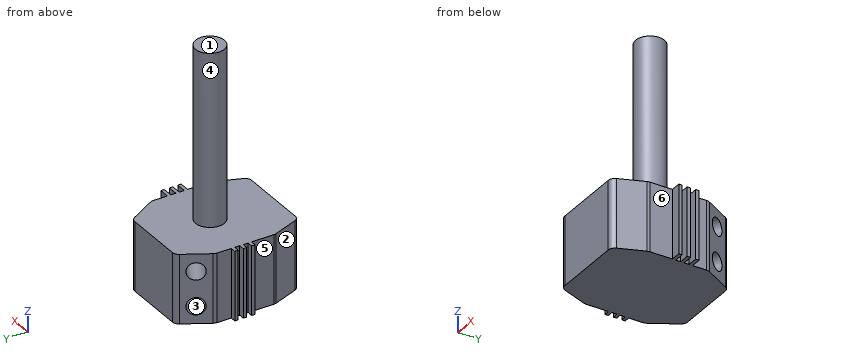
```python
from build123d import *

# Parameters (mm, degrees)
BOSS_EXTRUDE1_DEPTH = 20
SKETCH2_R           = 4.175
BOSS_EXTRUDE2_DEPTH = 50
SKETCH3_R           = 2.5
CUT_EXTRUDE1_DEPTH  = 20
SKETCH4_R           = 2.5
CUT_EXTRUDE2_DEPTH  = 20
SKETCH5_W           = 20
SKETCH5_H           = 1
BOSS_EXTRUDE3_DEPTH = 3


with BuildPart() as part:
    # Sketch1 → Boss-Extrude1 (new body)
    with BuildSketch(Plane.XY):
        with BuildLine():
            Line((7.995487969, -56.473761751), (-9.363697209, -56.473761751))
            ThreePointArc((-9.363697209, -56.473761751), (-10.367550845, -56.743941564), (-11.100183493, -57.481483874))
            Line((-11.100183493, -57.481483874), (-15.206075193, -64.666794349))
            ThreePointArc((-15.206075193, -64.666794349), (-15.402588207, -65.145736355), (-15.469588909, -65.659072225))
            Line((-15.469588909, -65.659072225), (-15.469588909, -82.177343211))
            ThreePointArc((-15.469588909, -82.177343211), (-15.435979311, -82.54245797), (-15.336280121, -82.895301369))
            Line((-15.336280121, -82.895301369), (-12.59092286, -90.03323025))
            ThreePointArc((-12.59092286, -90.03323025), (-11.856504513, -90.963895201), (-10.724231647, -91.315272091))
            Line((-10.724231647, -91.315272091), (9.356022407, -91.315272091))
            ThreePointArc((9.356022407, -91.315272091), (10.488295272, -90.963895201), (11.22271362, -90.03323025))
            Line((11.22271362, -90.03323025), (13.968070881, -82.895301369))
            ThreePointArc((13.968070881, -82.895301369), (14.067770071, -82.54245797), (14.101379669, -82.177343211))
            Line((14.101379669, -82.177343211), (14.101379669, -65.659072225))
            ThreePointArc((14.101379669, -65.659072225), (14.034378966, -65.145736355), (13.837865953, -64.666794349))
            Line((13.837865953, -64.666794349), (9.731974253, -57.481483874))
            ThreePointArc((9.731974253, -57.481483874), (8.999341605, -56.743941564), (7.995487969, -56.473761751))
        make_face()
    extrude(amount=BOSS_EXTRUDE1_DEPTH)

    # Sketch2 → Boss-Extrude2 (add)
    with BuildSketch(Plane.XY.offset(20)):
        with Locations(Location((-0.677787665, -72.858920612, 0), (0, 0, 180))):
            Circle(SKETCH2_R)
    extrude(amount=BOSS_EXTRUDE2_DEPTH)

    # Sketch3 → Cut-Extrude1 (cut)
    with BuildSketch(Plane(origin=(-17.424843232, -9.957053275, 0), x_dir=(0, 0, -1), z_dir=(0.868243142124459, 0.4961389383568344, 0))):
        with Locations(Location((-15, -59.074401838, 0), (0, 0, 90))):
            Circle(SKETCH3_R)
        with Locations(Location((-5, -59.074401838, 0), (0, 0, 90))):
            Circle(SKETCH3_R)
    extrude(amount=-CUT_EXTRUDE1_DEPTH, mode=Mode.SUBTRACT)

    # Sketch4 → Cut-Extrude2 (cut)
    with BuildSketch(Plane(origin=(16.393423958, -9.367670833, 0), x_dir=(0, 0, 1), z_dir=(-0.8682431421244587, 0.4961389383568347, 0))):
        with Locations(Location((5, -59.480800533, 0), (0, 0, 270))):
            Circle(SKETCH4_R)
        with Locations(Location((15, -59.480800533, 0), (0, 0, 270))):
            Circle(SKETCH4_R)
    extrude(amount=-CUT_EXTRUDE2_DEPTH, mode=Mode.SUBTRACT)

    # Sketch5 → Boss-Extrude3 (add)
    with BuildSketch(Plane(origin=(14.101379669, 0, 0), x_dir=(0, 0, -1), z_dir=(1, 0, 0))):
        with Locations((-10, -70.26948122)):
            Rectangle(SKETCH5_W, SKETCH5_H)
        with Locations((-10, -72.728796036)):
            Rectangle(SKETCH5_W, SKETCH5_H)
        with Locations((-10, -75.163517703)):
            Rectangle(SKETCH5_W, SKETCH5_H)
    boss_extrude3 = extrude(amount=BOSS_EXTRUDE3_DEPTH)

    # Mirror1: Boss-Extrude3 across plane
    add(boss_extrude3.mirror(Plane(origin=(0, 0, 0), x_dir=(0, 0, 1), z_dir=(1, 0, 0))))


solid = part.part
```
Geometry: final body of the model. Coordinates: model frame, mm. Face numbers are marked on the shaded views. A direction names the side the tool comes from. Coordinates: 2 decimals unless noted, no trailing zeros. Loops run counter-clockwise (first coordinate to the right, second up) from the corner with the lowest first, then second, coordinate; pieces in that order, holes last. Notation, with made-up numbers: M 12,42 L 19,42 A25 cw 19,61 Z; hole C 58.25,-29 d11. An arc over 180 degrees is marked long. Put each result on its own line as item: value.
(1) Cut plane B-B on x = 7. State how many separate pieces and enclosed holes the cut face has, then the cut area to 3 significant figures.
Answer sheet:
separate pieces: 1
enclosed holes: 2
area: 652 mm^2
(2) First-contact query: pin 1 (1.8 mm diameter, centred on x = -16.5, z = 7, fed in from -Y); pin 2 (10 mm diameter, centred on x = -6, z = 51, fed in from +Y); pin 3 (12 mm diameter, centred on x = 9, y = -85, fed in from +Z). Flat tips, straight axial feed; report the tip coordinate or a pass-through.
Answer sheet:
pin 1: stops at y = -75.66
pin 2: stops at y = -68.7
pin 3: stops at z = 20
(3) Material intervals for probe 1 along Y at (x, z) = (-5.5, 16.5); probe 2 along Z at (x, y) = (-3.5, -71.5); probe 3 along Z at (x, y) = (-13, -76), sorted ascending.
Answer sheet:
probe 1: y = -91.32 to -71.14, -68.88 to -67.67, -63.06 to -56.47
probe 2: z = 0 to 2.85, 7.15 to 12.85, 17.15 to 70
probe 3: z = 0 to 20
(4) Cut plane C-C on z = 25. Return the cut outline in (x, y) (3 decimals), then the cut area to 3 significant figures.
Answer sheet:
outline: C -0.678,-72.859 d8.35
area: 54.8 mm^2
(5) Access query for the marked faces 4, 5 and 6. Directions: +Z, -Z, +X, -X, +Y, -Y. A direction counts if a zero-diameter tool reaches every point of the face in a straight line with its end or side. Return the directions, or none.
Answer sheet:
face 4: +Z
face 5: +Z, -Z, -X, -Y
face 6: +Z, -Z, +X, -Y
(6) Cut plane A-A on y = -78. Return the cut outline in (x, z).
Answer sheet:
outline: M -15.47,0 L 14.1,0 L 14.1,20 L -15.47,20 Z
(7) Draft query along Z for the marked faces 1, 2 and 3. Return one class per face: pulls with the +Z half, pulls with the -Z half, needs draft (parallel to the pull), parting line crosses it, or undercut.
Answer sheet:
face 1: pulls with the +Z half
face 2: needs draft
face 3: undercut
